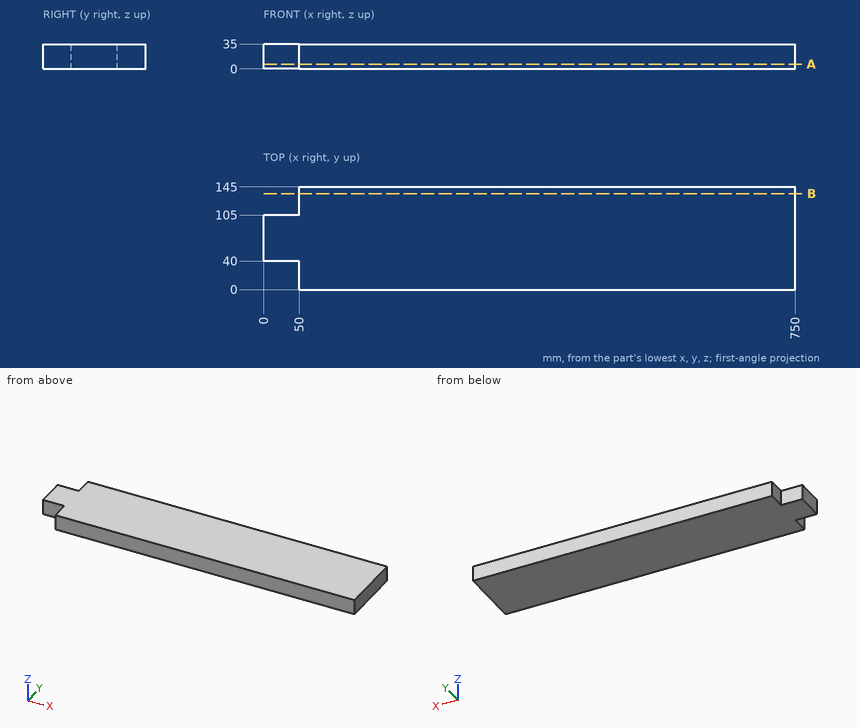
Geometry: see drawing. Coordinates: mm, zero at the bounding-box minimum. Give positions to 0.01 mm unless a question says otherwise; leave off trailing zeros. Order: outer loops, then holes, each group sorted by start corner. A loop starts at its lowest first (then second) coordinate and runs counter-clockwise, first axis right, second up. Notation, with made-up numbers: (78.5, 67.25) - (83.5, 67.25) arc R13 ccw to (83.5, 71.25) - close; hole circle Ø3 at (86.5, 4.5). An arc over 180 degrees is marked (long way). Use a Markdown table: item, result.
(1) Section query B-B (y = 135.5). Output: boundary loops of the cut face in (x, z).
Computed values:
| item | result |
|---|---|
| outline | (50, 0) - (750, 0) - (750, 35) - (50, 35) - close |
(2) Pin query (flat end, axial travel): pin 1 (1.5 mm diameter, centred on x = 123, y = 101.5, fed in from -Z); pin 2 (10.5 mm diameter, centred on y = 122.5, z = 18.5, fed in from -X). Return the tip coordinate at first contact, or that it passes through.
Computed values:
| item | result |
|---|---|
| pin 1 | stops at z = 0 |
| pin 2 | stops at x = 50 |
(3) Section query A-A (z = 6.5). Output: boundary loops of the cut face in (x, y), then the cut area to 3 significant figures.
Computed values:
| item | result |
|---|---|
| outline | (0, 40) - (50, 40) - (50, 0) - (750, 0) - (750, 145) - (50, 145) - (50, 105) - (0, 105) - close |
| area | 105,000 mm2 |
(4) Line query: line 1 (X direction, y = 113.5, z = 30.5); line 2 (Y direction, x = 48, z = 12). Output: solid intervals per line, ascending. Write a range as from..to.
Computed values:
| item | result |
|---|---|
| line 1 | x = 50..750 |
| line 2 | y = 40..105 |
